The figure shows three views and two pictorial views of one solid part (mm, origin at its lowest corner). Answer the questions. A direction names the side the tool comes from. Give positions to 0.01 mm unless a question says otherwise; leave off trailing zeros. Order: outer loops, then holes, each group sorted by start corner. A loop starts at its lowest first (then second) coordinate and runs counter-clockwise, first axis right, second up. Notation, with made-up numbers: (19, 34) -> (33, 34) arc R31 cw to (33, 71) -> close; hole circle Ø8 at (58, 53). An arc over 180 degrees is marked (long way). Use one line per item in the form item = value.
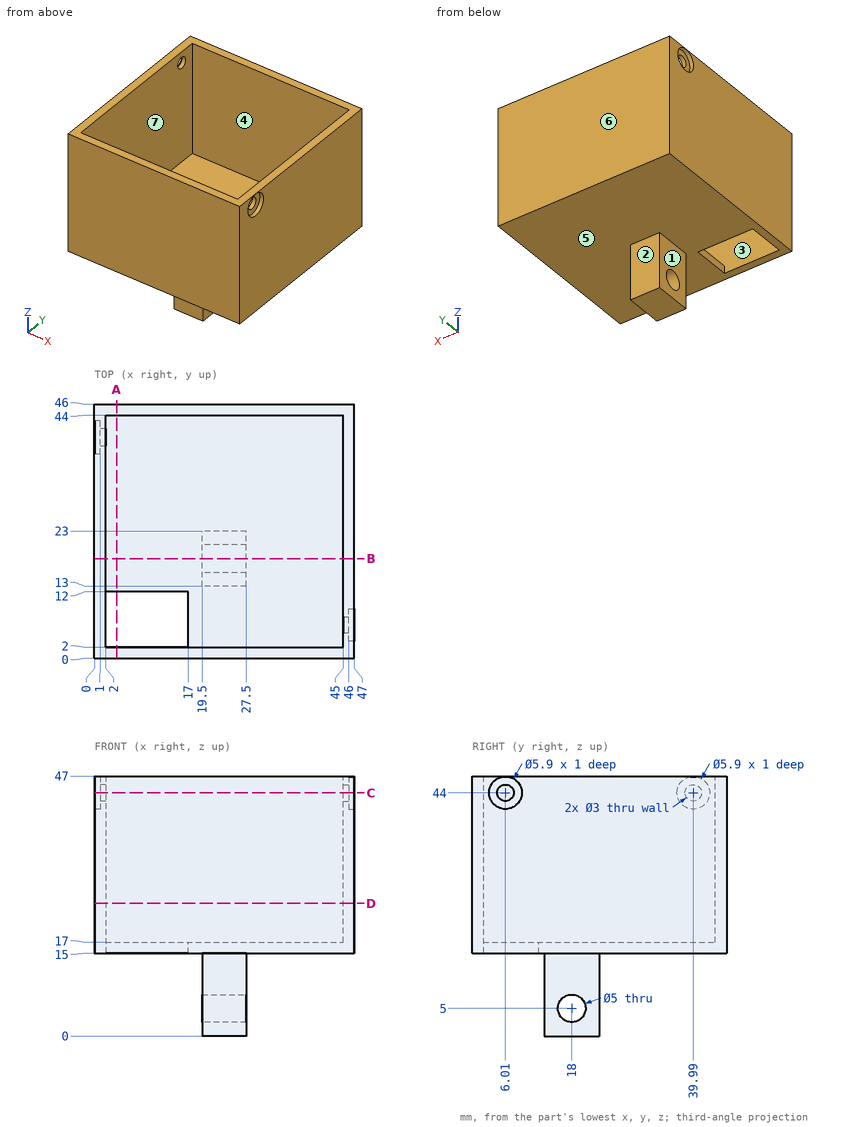
Item 1: Straight lines are drawn through the part: L1, parallel to X at y = 20, z = 26; L2, parallel to Y at x = 7, z = 39.5; L3, parallel to Z at x = 18, y = 20. For each, find the intervals that lie inside material, in ascending order. Write a range as from..to.
Checks:
L1 = 0..2, 45..47
L2 = 0..2, 44..46
L3 = 15..17
Item 2: The part is cut by section C-C on z = 44. Give the vertices of the cut face in (x, y).
Checks:
outline = (0, 0) -> (47, 0) -> (47, 3.06) -> (46, 3.06) -> (46, 4.51) -> (45, 4.51) -> (45, 2) -> (2, 2) -> (2, 38.49) -> (1, 38.49) -> (1, 37.04) -> (0, 37.04) -> close; (0, 42.94) -> (1, 42.94) -> (1, 41.49) -> (2, 41.49) -> (2, 44) -> (45, 44) -> (45, 7.51) -> (46, 7.51) -> (46, 8.96) -> (47, 8.96) -> (47, 46) -> (0, 46) -> close
Item 3: Given pin 1 Ø5 at (x, y) = (36, 26.5) entering from -Z; pin 2 Ø1.8 at (y, z) = (6.5, 42.5) entering from +X; pin 3 Ø5 at (y, z) = (32.5, 34) entering from -X; pin 4 Ø5 at (x, y) = (26.5, 6.5) entering from +Z, each flat-ended and moving along its own axis, determine where each tip first touches the part or whether it passes through.
Checks:
pin_1 = 15
pin_2 = 46
pin_3 = 0
pin_4 = 17
Item 4: Determine the mould class of the marked faces 4, 5, 6 and 7 for opening direction Y: +Y half, -Y half, draft (parallel to the pull), parting line (faces both ways), or undercut.
Checks:
face_4 = undercut
face_5 = draft
face_6 = +Y half
face_7 = undercut
Item 5: The part is cut by section A-A on x = 4. Give the vertices of the cut face in (y, z).
Checks:
outline = (0, 15) -> (2, 15) -> (2, 47) -> (0, 47) -> close; (12, 15) -> (46, 15) -> (46, 47) -> (44, 47) -> (44, 17) -> (12, 17) -> close
Item 6: The part is cut by section B-B on y = 18. Give the vertices of the cut face in (x, z).
Checks:
outline = (0, 15) -> (19.5, 15) -> (19.5, 7.5) -> (27.5, 7.5) -> (27.5, 15) -> (47, 15) -> (47, 47) -> (45, 47) -> (45, 17) -> (2, 17) -> (2, 47) -> (0, 47) -> close; (19.5, 0) -> (27.5, 0) -> (27.5, 2.5) -> (19.5, 2.5) -> close
Item 7: The part is cut by section D-D on z = 24. Give the vertices of the cut face in (x, y).
Checks:
outline = (0, 0) -> (47, 0) -> (47, 46) -> (0, 46) -> close; hole (2, 2) -> (45, 2) -> (45, 44) -> (2, 44) -> close
Item 8: Which of the six approach directions +Z, -Z, +X, -X, +Y, -Y give full straight-line access (tool end or side, diameter ignored) to the marked faces 1, 2 and 3?
Checks:
face_1 = -Z, -X, +Y, -Y
face_2 = -Z, +X, -X, +Y
face_3 = +Z
